Source: CAD feature listing. Evaluate the final solid. Frame: model axes, mm. A direction names the side the tool comes from. Round coordinates to 2 decimals unless told otherwise and drop trailing zeros. Loops run counter-clockwise (first coordinate to the right, second up) from the corner with the lowest first, then second, coordinate; pieces in that order, holes last. Notation, with made-up numbers: M -20,44 L 14,44 A38 ccw 14,82 Z; hole C -4.75,-35 d7. An arc over 180 degrees is marked long. Answer as a JSON object with one key per item and string values.
from build123d import *

# Parameters (mm, degrees)
SKETCH_1_W      = 250
SKETCH_1_H      = 120
EXTRUDE_1_DEPTH = 5
SKETCH_2_W      = 30
SKETCH_2_H      = 30
SKETCH_2_R      = 5
EXTRUDE_2_DEPTH = 5
FILLET_1_R      = 10


with BuildPart() as part:
    # Эскиз1 → Бобышка-Вытянуть1 (new body)
    with BuildSketch(Plane(origin=(0, 0, 0), x_dir=(1, 0, 0), z_dir=(0, 1, 0))):
        Rectangle(SKETCH_1_W, SKETCH_1_H)
    extrude(amount=EXTRUDE_1_DEPTH)


with BuildPart() as body_2:
    # Эскиз2 → Бобышка-Вытянуть2 (new body)
    with BuildSketch(Plane(origin=(0, 0, 0), x_dir=(1, 0, 0), z_dir=(0, 1, 0))):
        with Locations((-80, 75)):
            Rectangle(SKETCH_2_W, SKETCH_2_H)
        with Locations(Location((-80, 75, 0), (0, 0, 270))):
            Circle(SKETCH_2_R, mode=Mode.SUBTRACT)
    extrude(amount=EXTRUDE_2_DEPTH)

    # Скругление1
    fillet_1_edges = [body_2.edges().sort_by_distance(p)[0] for p in [
        (-95, 2.5, -90),
        (-65, 2.5, -90),
    ]]
    fillet(fillet_1_edges, radius=FILLET_1_R)


with BuildPart() as body_3:
    # Зеркальное отражение1: mirrored copy
    add(body_2.part.mirror(Plane(origin=(0, 0, 0), x_dir=(0, 0, 1), z_dir=(1, 0, 0))))


with BuildPart() as body_4:
    # Зеркальное отражение3: mirrored copy
    add(body_2.part.mirror(Plane.XY))


with BuildPart() as body_5:
    # Mirror 3 2: mirrored copy
    add(body_3.part.mirror(Plane.XY))


with BuildPart() as part_1:
    add(part.part)

    # Combine 1: union body 4, body 3, body 2, body 5
    add(body_4.part)
    add(body_3.part)
    add(body_2.part)
    add(body_5.part)


solid = part_1.part
Item 1: Access query for faces 4 (the flat face through (-95, 2, 70)), 5 (the cylindrical face through (68.01, 2.54, -87.15)), 6 (the flat face through (110, 2, 60)), 7 (the flat face through (-110, 2, -60)), 8 (the cylindrical face through (-68.01, 2.54, 87.15)). Directions: +Z, -Z, +X, -X, +Y, -Y. A direction counts if a zero-diameter tool reaches every point of the face in a straight line with its end or side. Return the directions, or none.
Answer sheet:
{"face 4": "+Z, -X, +Y, -Y", "face 5": "-Z, +Y, -Y", "face 6": "+Z, +X, +Y, -Y", "face 7": "-Z, -X, +Y, -Y", "face 8": "+Z, +Y, -Y"}
Item 2: Pull-direction query (Z, two-part tool) for faces 1 (the flat face through (-2, 0, -1)), 2 (the cylindrical face through (92.15, 2.54, -86.99)), 3 (the cylindrical face through (-81.915, 2.465, 70.381)); classes: pulls with the +Z half, pulls with the -Z half, needs draft (parallel to the pull), parting line crosses it, or undercut.
Answer sheet:
{"face 1": "needs draft", "face 2": "pulls with the -Z half", "face 3": "undercut"}
Item 3: Section D-D on x = -14. Return the cut outline in (y, z).
Answer sheet:
{"outline": "M 0,-60 L 5,-60 L 5,60 L 0,60 Z"}
Item 4: Contact query for flat-ended pins moving along their axis: pin 1 Ø1.5 at (y, z) = (2, -70.5) entering from -X; pin 2 Ø1.5 at (x, y) = (104, 3) entering from -Z; pin 3 Ø2.5 at (y, z) = (2, -68.5) entering from +X. Output: stop coordinate, or through.
Answer sheet:
{"pin 1": "stops at x = -95", "pin 2": "stops at z = -60", "pin 3": "stops at x = 95"}
Item 5: Section C-C on y = 1.6. Give the number of separate pieces and of enclosed holes in the cut face, then the cut area to 3 significant figures.
Answer sheet:
{"separate pieces": "1", "enclosed holes": "4", "area": "33,100 mm²"}
Item 6: Section A-A on x = -80. Return the cut outline in (y, z).
Answer sheet:
{"outline": "M 0,-90 L 5,-90 L 5,-80 L 0,-80 Z; M 0,-70 L 5,-70 L 5,70 L 0,70 Z; M 0,80 L 5,80 L 5,90 L 0,90 Z"}
Item 7: Line query: probe 1 along Z at (x, y) = (80, 1.6); probe 2 along X at (y, z) = (3.8, -75); probe 3 along Z at (x, y) = (100.5, 4.4). Output: solid intervals per line, ascending. Write a range as from..to.
Answer sheet:
{"probe 1": "z = -90..-80, -70..70, 80..90", "probe 2": "x = -95..-85, -75..-65, 65..75, 85..95", "probe 3": "z = -60..60"}
Item 8: Section B-B on z = -75. Return the cut outline in (x, y), then the cut area to 3 significant figures.
Answer sheet:
{"outline": "M -95,0 L -85,0 L -85,5 L -95,5 Z; M -75,0 L -65,0 L -65,5 L -75,5 Z; M 65,0 L 75,0 L 75,5 L 65,5 Z; M 85,0 L 95,0 L 95,5 L 85,5 Z", "area": "200 mm²"}
